```python
from build123d import *
from build123d.topology import SkipClean

# Parameters (mm, degrees)
SKETCH1_R           = 225
BOSS_EXTRUDE1_DEPTH = 500
SKETCH2_R           = 295
BOSS_EXTRUDE2_DEPTH = 135
FILLET1_R           = 25
BOSS_EXTRUDE3_DEPTH = 274
SKETCH7_R           = 87.5
CUT_EXTRUDE1_DEPTH  = 548
SKETCH8_R           = 295
BOSS_EXTRUDE4_DEPTH = 135


with BuildPart() as part:
    # Sketch1 → Boss-Extrude1 (new body)
    with BuildSketch(Plane.XY):
        Circle(SKETCH1_R)
    extrude(amount=-BOSS_EXTRUDE1_DEPTH)

    # Sketch2 → Boss-Extrude2 (add)
    with BuildSketch(Plane(origin=(0, 0, -500), x_dir=(-1, 0, 0), z_dir=(0, 0, -1))):
        Circle(SKETCH2_R)
    extrude(amount=BOSS_EXTRUDE2_DEPTH)

    # Fillet1
    fillet1_edges = [part.edges().sort_by_distance(p)[0] for p in [
        (-225, 0, 0),
        (-225, 0, -500),
    ]]
    fillet(fillet1_edges, radius=FILLET1_R)

    # Sketch5 → Boss-Extrude3 (add, symmetric)
    with BuildSketch(Plane(origin=(0, 0, 0), x_dir=(1, 0, 0), z_dir=(0, 1, 0))):
        with BuildLine():
            Line((0, 525.936531369), (-80, 525.936531369))
            ThreePointArc((-80, 525.936531369), (-362.842712475, 643.093818894), (-480, 925.936531369))
            Line((-480, 925.936531369), (-480, 1250))
            Line((-480, 1250), (-400, 1250))
            Line((-400, 1250), (-400, 925.936531369))
            ThreePointArc((-400, 925.936531369), (-306.27416998, 699.662361389), (-80, 605.936531369))
            Line((-80, 605.936531369), (0, 605.936531369))
            Line((0, 605.936531369), (0, 525.936531369))
        make_face()
    boss_extrude3 = extrude(amount=BOSS_EXTRUDE3_DEPTH, both=True)

    # Sketch7 → Cut-Extrude1 (cut)
    with BuildSketch(Plane(origin=(0, 0, 0), x_dir=(0, 0, -1), z_dir=(1, 0, 0))):
        with Locations((1125, 0)):
            Circle(SKETCH7_R)
        with BuildLine():
            Line((1049.174263404, 219.16283358), (203.039318936, 293.190049034))
            Line((203.039318936, 293.190049034), (290.021270447, 513.829798209))
            Line((290.021270447, 513.829798209), (1323.371387979, 627.428253954))
            Line((1323.371387979, 627.428253954), (2049.606507286, -712.594868551))
            Line((2049.606507286, -712.594868551), (1049.174263404, -1026.824287114))
            Line((1049.174263404, -1026.824287114), (203.039318936, -293.190049034))
            Line((203.039318936, -293.190049034), (1049.174263404, -219.16283358))
            ThreePointArc((1049.174263404, -219.16283358), (1250, 0), (1049.174263404, 219.16283358))
        make_face()
    cut_extrude1 = extrude(amount=-CUT_EXTRUDE1_DEPTH, mode=Mode.SUBTRACT)

    # Sketch8 → Boss-Extrude4 (add)
    with BuildSketch(Plane.XY.offset(-500)):
        with Locations(Location((0, 0, 0), (0, 0, 243.787314881))):
            Circle(SKETCH8_R)
    boss_extrude4 = extrude(amount=-BOSS_EXTRUDE4_DEPTH)

    # Mirror3: Boss-Extrude3, Cut-Extrude1, Boss-Extrude4 across plane
    with SkipClean():  # the faces are left unmerged after this step: merging them gives an invalid solid
        add(boss_extrude3.mirror(Plane(origin=(0, 0, 0), x_dir=(0, 0, 1), z_dir=(1, 0, 0))))
        add(cut_extrude1.mirror(Plane(origin=(0, 0, 0), x_dir=(0, 0, 1), z_dir=(1, 0, 0))), mode=Mode.SUBTRACT)
        add(boss_extrude4.mirror(Plane(origin=(0, 0, 0), x_dir=(0, 0, 1), z_dir=(1, 0, 0))))
    add(part.part.scale(1), mode=Mode.REPLACE)  # the faces are merged on a copy


solid = part.part
```
Can you work these out from the model? Positions are in its coordinate system, mm. A direction names the side the tool comes from. Give positions to 0.01 mm unless a question says otherwise; leave off trailing zeros. Loops run counter-clockwise (first coordinate to the right, second up) from the corner with the lowest first, then second, coordinate; pieces in that order, holes last. Notation, with made-up numbers: M 55,-7.75 L 66,-7.75 A28 cw 66,16.25 Z; hole C 0.5,-32 d7. An arc over 180 degrees is marked long. Use one line per item in the form item = value. Start each with the question number.
(1) I want a section at B-B, the plane z = -654. Write out the boundary of the cut face in (x, y).
(2) I want a section at A-A, the plane z = -1155. Write out the boundary of the cut face in (x, y), and give its area (3 significant figures).
(3) I want a section at C-C, the plane y = 65. State how many separate pieces and enclosed holes the cut face has, and give its area (3 significant figures).
(4) Thinking about a two-plate mould opening in Y: for faces 4 (the flat face through (400, 3, -1018)), 5 (the flat face through (-369.094, 245.177, -751.834)), 6 (the cylindrical face through (-224.782, 9.893, -246.85)), 7 (the cylindrical face through (-439.44, 3.847, -1037.585)), which applies, released by +Y, released by -Y, zero draft, split by the parting line, or undercut?
(5) I want a section at D-D, the plane x = -420. Write out the boundary of the cut face in (y, z).
(6) I'm going to push flat-ended pins straight in: P1, Ø2, axis at y = -144.5, z = -803, coming from the -X side; P2, Ø22, axis at x = -92, y = 288, coming from the +Z side; P3, Ø3, axis at x = -79.5, z = -406.5, coming from the +Y side. Where does each tip first touch, or does it pass through?
(7) On a 3-axis mill with a long thin cutter (end or side, diameter ignored), from which of +Z, -Z, +X, -X, +Y, -Y can I reach the whole of each face in a straight line? I mean faces 1 (the flat face through (-356.14, -245.39, -749.41)), 2 (the flat face through (369.094, 245.177, -751.834)), 3 (the flat face through (356.14, -245.39, -749.41)). Say none if no direction works.
(8) Please list where these lines run through material, in increasing order: line 1 (Z direction, x = 164, y = -71); line 2 (Y direction, x = 443.5, z = -1125); line 3 (Z direction, x = 186.5, y = 187).
Worked out:
q1.outline = M -373.34,-253.74 L -248.67,-253.74 L -248.67,253.74 L -373.34,253.74 Z; M 248.67,-253.74 L 373.34,-253.74 L 373.34,253.74 L 248.67,253.74 Z
q2.outline = M -480,-181.04 L -400,-181.04 L -400,-82.2 L -480,-82.2 Z; M -480,82.2 L -400,82.2 L -400,181.04 L -480,181.04 Z; M 400,-181.04 L 480,-181.04 L 480,-82.2 L 400,-82.2 Z; M 400,82.2 L 480,82.2 L 480,181.04 L 400,181.04 Z
q2.area = 31,600 mm²
q3.separate_pieces = 3
q3.enclosed_holes = 0
q3.area = 383,000 mm²
q4.face_4 = zero draft
q4.face_5 = released by +Y
q4.face_6 = split by the parting line
q4.face_7 = undercut
q5.outline = M -248.38,-715.22 L -219.16,-1049.17 A220 ccw 219.16,-1049.17 L 248.38,-715.22 Z; hole C 0,-1125 d175
q6.P1 = -460.96
q6.P2 = -500
q6.P3 = 211.05
q7.face_1 = -Z, -X, -Y
q7.face_2 = -Z, +X, +Y
q7.face_3 = -Z, +X, -Y
q8.line_1 = -635 to 0
q8.line_2 = -198.43 to -87.5, 87.5 to 198.43
q8.line_3 = -635 to -500
